Geometry: final body of the model. Coordinates: model frame, mm. Face numbers are marked on the shaded views. A direction names the side the tool comes from. Round coordinates to 2 decimals unless told otherwise and drop trailing zeros. Order: outer loops, then holes, each group sorted by start corner. A loop starts at its lowest first (then second) coordinate and runs counter-clockwise, first axis right, second up. Notation, with made-up numbers: M 36.25,-2 L 80.25,-2 A21 cw 80.25,3 Z; hole C 67,44.5 d4. An arc over 180 degrees is marked long. Return JSON: item names as keys, results as strings. Group by question number.
Q1. Mould query, pull axis Z, two halves, no side actions, for the marked faces 3, 4 and 5. Classes: released by +Z, released by -Z, zero draft, split by the parting line, or undercut.
Q2. Ray query, probe 1 along X at (y, z) = (-0.5, 0); probe 2 along X at (y, z) = (-5.25, -4.75); probe 3 along Z at (x, y) = (-3, -3.25). Return the intervals inside material, ascending.
Q3. Cut plane A-A on y = -1. Output: boundary loops of the cut face in (x, z).
Q4. Cut plane C-C on y = -4.5. Output: boundary loops of the cut face in (x, z) (3 decimals), and give its area (3 significant figures).
Q5. Cut plane D-D on z = 0. Output: boundary loops of the cut face in (x, y) (3 decimals).
Q6. Access query for the marked faces 1 and 2. Directions: +Z, -Z, +X, -X, +Y, -Y. A direction counts if a zero-diameter tool reaches every point of the face in a straight line with its end or side. Return the directions, or none.
Q7. Contact query for flat-ended pins moving along their axis: pin 1 (1.3 mm diameter, centred on x = 2.5, y = -4.5, fed in from +Z); pin 2 (1 mm diameter, centred on x = -9, y = -3.5, fed in from +Z); pin 3 (1.3 mm diameter, centred on x = -3, y = -2.5, fed in from -Z). Output: stop coordinate, or through.
Q8. Cut plane B-B on x = 0. Output: boundary loops of the cut face in (y, z) (3 decimals).
```python
from build123d import *

# Parameters (mm, degrees)
F0_R     = 10
F1_DEPTH = 6.35
F4_DEPTH = 23
F5_DEPTH = 3
F6_DEPTH = 25


# Not quite as in the source:
# - a feature names something its author has since deleted; it is built from what else it names


with BuildPart() as f1:
    # F0 (on Front) → F1 (new body)
    with BuildSketch(Plane.XZ):
        Circle(F0_R)
        Polygon((-3.75, -5.5), (-3.75, -1), (-3.75, 1), (-3.75, 5.5), (-1.75, 5.5), (-1.75, 1), (1.75, 1), (1.75, 5.5), (3.75, 5.5), (3.75, 1), (3.75, -1), (3.75, -5.5), (1.75, -5.5), (1.75, -1), (-1.75, -1), (-1.75, -5.5), align=None, mode=Mode.SUBTRACT)
    extrude(amount=F1_DEPTH)

    # F3 (on offset) → F4 (join)
    with BuildSketch(Plane.YZ.offset(-9.7)):
        Polygon((-1.375, -2.2), (-1.375, 0), (-1.375, 2.2), (-2.575, 2.2), (-2.575, 1.0935393064), (-3.775, 1.0935393064), (-3.775, 2.2), (-4.975, 2.2), (-4.975, -2.2), (-3.775, -2.2), (-3.775, -0.9002136735), (-2.575, -0.9002136735), (-2.575, -2.2), align=None)
    extrude(amount=F4_DEPTH)

    # F3 (on offset) → F5 (cut)
    with BuildSketch(Plane.YZ.offset(-9.7)):
        Polygon((-1.375, -2.2), (-1.375, 0), (-1.375, 2.2), (-2.575, 2.2), (-2.575, 1.0935393064), (-3.775, 1.0935393064), (-3.775, 2.2), (-4.975, 2.2), (-4.975, -2.2), (-3.775, -2.2), (-3.775, -0.9002136735), (-2.575, -0.9002136735), (-2.575, -2.2), align=None)
    extrude(amount=F5_DEPTH, mode=Mode.SUBTRACT)

    # F3 (on offset) → F6 (cut)
    with BuildSketch(Plane.YZ.offset(-9.7)):
        Polygon((-1.375, -2.2), (-1.375, 0), (-1.375, 2.2), (-2.575, 2.2), (-2.575, 1.0935393064), (-3.775, 1.0935393064), (-3.775, 2.2), (-4.975, 2.2), (-4.975, -2.2), (-3.775, -2.2), (-3.775, -0.9002136735), (-2.575, -0.9002136735), (-2.575, -2.2), align=None)
    extrude(amount=-F6_DEPTH, mode=Mode.SUBTRACT)


solid = f1.part
```
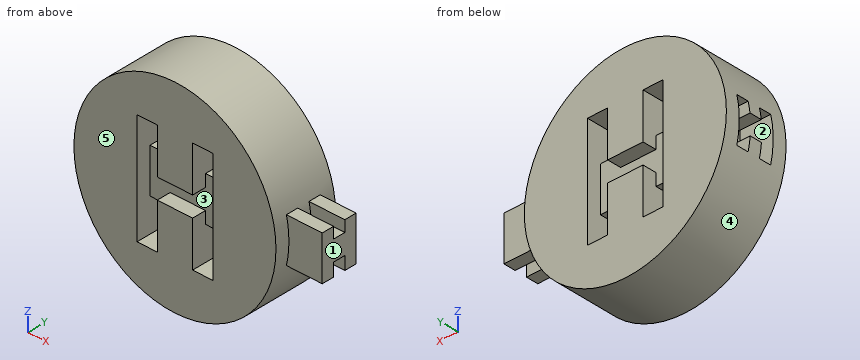
Result sheet:
{
 "1": {"face 3": "undercut", "face 4": "split by the parting line", "face 5": "zero draft"},
 "2": {"probe 1": "x = -10 to -3.75, 3.75 to 10", "probe 2": "x = -8.8 to -3.75, -1.75 to 1.75, 3.75 to 8.8", "probe 3": "z = -9.54 to -5.5, -0.9 to 1.09, 5.5 to 9.54"},
 "3": {"outline": "C 0,0 d20; hole M -3.75,-5.5 L -1.75,-5.5 L -1.75,-1 L 1.75,-1 L 1.75,-5.5 L 3.75,-5.5 L 3.75,5.5 L 1.75,5.5 L 1.75,1 L -1.75,1 L -1.75,5.5 L -3.75,5.5 Z"},
 "4": {"outline": "M -9.755,-2.2 A10 ccw 9.755,-2.2 L 13.3,-2.2 L 13.3,2.2 L 9.755,2.2 A10 ccw -9.755,2.2 L -6.7,2.2 L -6.7,-2.2 Z; hole M -3.75,-5.5 L -1.75,-5.5 L -1.75,-2.2 L -3.75,-2.2 Z; hole M -3.75,2.2 L -1.75,2.2 L -1.75,5.5 L -3.75,5.5 Z; hole M 1.75,-5.5 L 3.75,-5.5 L 3.75,-2.2 L 1.75,-2.2 Z; hole M 1.75,2.2 L 3.75,2.2 L 3.75,5.5 L 1.75,5.5 Z", "area": "288 mm²"},
 "5": {"outline": "M -10,-6.35 L -3.75,-6.35 L -3.75,-4.975 L 3.75,-4.975 L 3.75,-6.35 L 10,-6.35 L 10,-4.975 L 13.3,-4.975 L 13.3,-1.375 L 10,-1.375 L 10,0 L 3.75,0 L 3.75,-1.375 L -3.75,-1.375 L -3.75,0 L -10,0 L -10,-1.375 L -6.7,-1.375 L -6.7,-4.975 L -10,-4.975 Z"},
 "6": {"face 1": "+Z, -Z, +X, +Y, -Y", "face 2": "-X"},
 "7": {"pin 1": "stops at z = 9.83", "pin 2": "stops at z = 5.27", "pin 3": "stops at z = -9.72"},
 "8": {"outline": "M -6.35,-10 L 0,-10 L 0,-1 L -1.375,-1 L -1.375,1 L 0,1 L 0,10 L -6.35,10 L -6.35,1 L -4.975,1 L -4.975,-1 L -6.35,-1 Z; hole M -3.775,-1 L -2.575,-1 L -2.575,-0.9 L -3.775,-0.9 Z"}
}
